Check sheet for the drawn part. Datum: minimum x, y, z corner. Units: mm. Round coordinates to 2 decimals unless told otherwise and drop trailing zeros. Write each loop counter-clockwise with the first axis right and the second up, starting at its lowest first coordinate (ties: lowest second). Pieces come first, ordered by that corner, then holes.
Item 1: Cross-section at B-B on z = 118. Enter the section's corners in (x, y).
Item 2: Cross-section at D-D on x = 201. Enter the section's corners in (y, z).
Item 3: Cross-section at C-C on y = 3.2. Enter the section's corners in (x, z).
Item 4: Cross-section at A-A on x = 265.5. Enter the section's corners in (y, z).
Item 5: Material ranges on line 1 (Z direction, x = 267.5, y = 2.55); line 2 (Z direction, x = 243, y = 0.85); line 3 (Z direction, x = 160, y = 0.4), recorded low to high.
Item 6: Go/stop test with flat-tipped pins: pin 1 Ø2 at (x, y) = (286.5, 1.5) entering from -Z; pin 2 Ø2 at (y, z) = (1.5, 87.5) entering from +X. Record where each tip stops, or that it passes through.
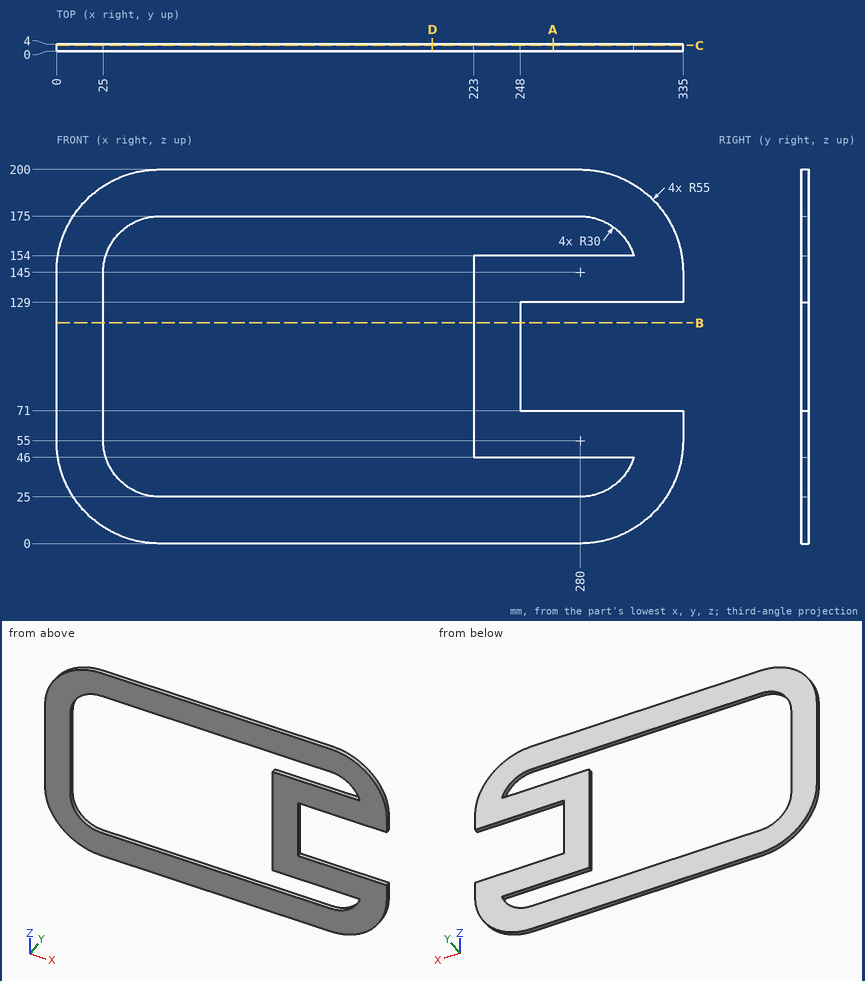
Response values:
1. outline: (0, 0) - (25, 0) - (25, 4) - (0, 4) - close; (223, 0) - (248, 0) - (248, 4) - (223, 4) - close
2. outline: (0, 0) - (4, 0) - (4, 25) - (0, 25) - close; (0, 175) - (4, 175) - (4, 200) - (0, 200) - close
3. outline: (0, 55) arc R55 ccw to (55, 0) - (280, 0) arc R55 ccw to (335, 55) - (335, 71) - (248, 71) - (248, 129) - (335, 129) - (335, 145) arc R55 ccw to (280, 200) - (55, 200) arc R55 ccw to (0, 145) - close; hole (25, 55) arc R30 ccw to (55, 25) - (280, 25) arc R30 ccw to (308.62, 46) - (223, 46) - (223, 154) - (308.62, 154) arc R30 ccw to (280, 175) - (55, 175) arc R30 ccw to (25, 145) - close
4. outline: (0, 0) - (4, 0) - (4, 25) - (0, 25) - close; (0, 46) - (4, 46) - (4, 71) - (0, 71) - close; (0, 129) - (4, 129) - (4, 154) - (0, 154) - close; (0, 175) - (4, 175) - (4, 200) - (0, 200) - close
5. line 1: z = 0 to 25, 46 to 71, 129 to 154, 175 to 200
5. line 2: z = 0 to 25, 46 to 154, 175 to 200
5. line 3: z = 0 to 25, 175 to 200
6. pin 1: stops at z = 0.28
6. pin 2: stops at x = 248
